The model under review builds one solid part; all positions refer to its coordinate system, in mm. A direction names the side the tool comes from. Round coordinates to 2 decimals unless told otherwise and drop trailing zeros. Order: outer loops, then holes, each group sorted by start corner. A loop starts at its lowest first (then second) coordinate and runs counter-clockwise, first axis right, second up.
1) To check wall thickness, follow L1, parallel to Z at x = 0, y = 93.5; L2, parallel to X at y = 25.5, z = 2.25. State the ranges of each line that lie inside material, in increasing order.
2) Mouldability with a two-part tool opening along Z and no side actions: class faces 1 (the face through (4.1, 49.3, -4.14)), 2 (the face through (-0.36, 78.96, -0.08)), 3 (the face through (0.1, 100, 2.3)) as pulls with the +Z half, pulls with the -Z half, needs draft (parallel to the pull), parting line crosses it, or undercut.
3) Consider section C-C (z = -3). Give the boundary of the cut face in (x, y).
4) Clearance check with flat-ended pins moving along their axes: P1, Ø3.5, axis at x = 0, z = 0, coming from the +Y side; P2, Ø2.5, axis at x = 0, z = 0, coming from the -Y side. State where each tip first meets the part, or that it passes through.
5) Machinability: for faces 4 (the face through (5, 49, 0)), 5 (the face through (-0.631, 89.86, 2.003)), 6 (the face through (-0.631, 10.14, -2.003)), which of the approach directions +Z, -Z, +X, -X, +Y, -Y give a long, thin tool a straight path to every point of the face, cutting with its end or side? Answer none if there is none.
6) Consider section D-D (x = -3.5). Give the boundary of the cut face in (y, z).
7) Consider section A-A (y = 93.5). Give the boundary of the cut face in (x, z), then the cut area to 3 significant figures.
8) Consider section B-B (y = 45.5). Give the boundary of the cut face in (x, z).
Autodesk Inventor part; units mm, degrees
ref_plane "YZ Plane" through (0, 0, 0) normal (1, 0, 0) x (0, 1, 0)
ref_plane "XZ Plane" through (0, 0, 0) normal (0, 1, 0) x (-1, 0, 0)
ref_plane "XY Plane" through (0, 0, 0) normal (0, 0, 1) x (1, 0, 0)
sketch "Boceto1" plane through (0, 0, 0) normal (0, 1, 0) x (-1, 0, 0)
  line L0 (-2, -5) -> (2, -5)
  line L1 (5, -2) -> (5, 2)
  line L2 (2, 5) -> (-2, 5)
  line L3 (-5, 2) -> (-5, -2)
  line L4 (-5, -5) -> (5, 5) construction
  line L5 (5, -5) -> (-5, 5) construction
  arc A0 (5, 2) -> (2, 5) centre (2, 2) ccw
  arc A1 (2, -5) -> (5, -2) centre (2, -2) ccw
  arc A2 (-5, -2) -> (-2, -5) centre (-2, -2) ccw
  arc A3 (-2, 5) -> (-5, 2) centre (-2, 2) ccw
  point P0 (0, 0)
  dimension "d0" = 10
  dimension "d1" = 10
  dimension "d2" = 3
extrude "Extrusión1" add sketch "Boceto1" along normal blind 100
sketch "Boceto2" plane through (0, 100, 0) normal (0, 1, 0) x (1, 0, 0)
  line L0 (2, 5) -> (-2, 5)
  line L1 (5, -2) -> (5, 2)
  point P0 (0, 0)
  point P1 (0, 0)
  dimension "d5" = 5
  dimension "d6" = 5
hole "Agujero1" at (0, 100, 0) direction (0, -1, 0) diameter 4.2 depth 20 tip angle 118
sketch "Boceto3" plane through (0, 0, 0) normal (0, -1, 0) x (1, 0, 0)
  line L0 (5, 2) -> (5, -2)
  line L1 (-2, 5) -> (2, 5)
  point P0 (0, 0)
  point P1 (0, 0)
  dimension "d14" = 5
  dimension "d15" = 5
hole "Agujero2" at (0, 0, 0) direction (0, 1, 0) diameter 4.2 depth 20 tip angle 118
properties part number "Columna"
Answer below:
1. L1: z = -5 to -2.1, 2.1 to 5
1. L2: x = -4.99 to 4.99
2. face 1: pulls with the -Z half
2. face 2: undercut
2. face 3: needs draft
3. outline: (-4.83, 0) - (4.83, 0) - (4.83, 100) - (-4.83, 100) - close
4. P1: stops at y = 79.79
4. P2: stops at y = 20.51
5. face 4: +Z, -Z, +X, +Y, -Y
5. face 5: +Y
5. face 6: -Y
6. outline: (0, -4.6) - (100, -4.6) - (100, 4.6) - (0, 4.6) - close
7. outline: (-5, -2) arc R3 ccw to (-2, -5) - (2, -5) arc R3 ccw to (5, -2) - (5, 2) arc R3 ccw to (2, 5) - (-2, 5) arc R3 ccw to (-5, 2) - close; hole circle Ø4.2 at (0, 0)
7. area: 78.4 mm2
8. outline: (-5, -2) arc R3 ccw to (-2, -5) - (2, -5) arc R3 ccw to (5, -2) - (5, 2) arc R3 ccw to (2, 5) - (-2, 5) arc R3 ccw to (-5, 2) - close
